Part model, mm, in its own coordinate system. Face numbers are marked on the shaded views. A direction names the side the tool comes from. Give positions to 0.01 mm unless a question says otherwise; leave off trailing zeros. Write each loop counter-clockwise with the first axis right and the second up, starting at its lowest first coordinate (ties: lowest second). Pieces come first, ordered by that corner, then holes.
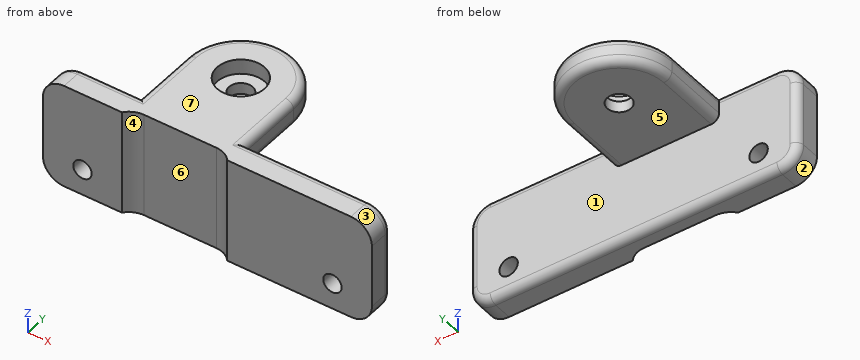
from build123d import *

# Parameters (mm, degrees)
SKETCH2_W                               = 125
SKETCH2_H                               = 40
BOSS_EXTRUDE1_DEPTH                     = 10
BOSS_EXTRUDE2_DEPTH                     = 10
SKETCH4_W                               = 40
SKETCH4_H                               = 3
CUT_EXTRUDE1_DEPTH                      = 80
CBORE_FOR_M8_HEX_HEAD_BOLT1_D           = 9
CBORE_FOR_M8_HEX_HEAD_BOLT1_CBORE_D     = 18.01
CBORE_FOR_M8_HEX_HEAD_BOLT1_CBORE_DEPTH = 5.68
FILLET2_R                               = 8
FILLET3_R                               = 3
F_7_0_7_DIAMETER_HOLE1_D                = 7


with BuildPart() as part:
    # Sketch2 → Boss-Extrude1 (new body)
    with BuildSketch(Plane(origin=(0, 0, 0), x_dir=(1, 0, 0), z_dir=(0, 1, 0))):
        with Locations((62.5, 20)):
            Rectangle(SKETCH2_W, SKETCH2_H)
    extrude(amount=BOSS_EXTRUDE1_DEPTH)

    # Sketch3 → Boss-Extrude2 (add)
    with BuildSketch(Plane.XY):
        with BuildLine():
            Line((30, 35), (30, 0))
            Line((30, 0), (70, 0))
            Line((70, 0), (70, 35))
            ThreePointArc((70, 35), (50, 55), (30, 35))
        make_face()
    extrude(amount=-BOSS_EXTRUDE2_DEPTH)

    # Sketch4 → Cut-Extrude1 (cut)
    with BuildSketch(Plane.XY):
        with Locations((50, 1.5)):
            Rectangle(SKETCH4_W, SKETCH4_H)
    extrude(amount=-CUT_EXTRUDE1_DEPTH, mode=Mode.SUBTRACT)

    # CBORE for M8 Hex Head Bolt1 (through all)
    with Locations(Plane(origin=(50, 35, 0), x_dir=(1, 0, 0), z_dir=(0, 0, 1))):
        with Locations((0, 0)):
            CounterBoreHole(CBORE_FOR_M8_HEX_HEAD_BOLT1_D / 2, CBORE_FOR_M8_HEX_HEAD_BOLT1_CBORE_D / 2, CBORE_FOR_M8_HEX_HEAD_BOLT1_CBORE_DEPTH)

    # Fillet2
    # the kernel refuses this fillet: 8 mm, written as the material it adds along each edge
    with BuildSketch(Plane(origin=(70, 3, 0), x_dir=(-1, 0, 0), z_dir=(0, 0, -1))) as fillet2_piece_1:
        with BuildLine():
            CenterArc((6.244997998, -8), FILLET2_R, 90, 51.317812547)
            Line((0, -3), (0, 0))
            Line((0, 0), (6.244997998, 0))
        make_face()
    extrude(amount=40)
    with BuildSketch(Plane(origin=(30, 3, 0), x_dir=(0, -1, 0), z_dir=(0, 0, -1))) as fillet2_piece_2:
        with BuildLine():
            CenterArc((8, -6.244997998), FILLET2_R, 128.682187453, 51.317812547)
            Line((0, -6.244997998), (0, 0))
            Line((0, 0), (3, 0))
        make_face()
    extrude(amount=40)
    # the kernel refuses this fillet: 8 mm, written as the material it takes off along each edge
    with BuildSketch(Plane(origin=(125, -20, 0), x_dir=(-1, 0, 0), z_dir=(0, 1, 0)), Plane(origin=(125, -20, -40), x_dir=(0, 0, 1), z_dir=(0, 1, 0))) as fillet2_2_piece_1:
        with BuildLine():
            CenterArc((FILLET2_R, -FILLET2_R), FILLET2_R, 90, 90)
            Line((0, -FILLET2_R), (0, 0))
            Line((0, 0), (FILLET2_R, 0))
        make_face()
    extrude(amount=50, mode=Mode.SUBTRACT)
    with BuildSketch(Plane(origin=(0, -20, -40), x_dir=(0, 0, 1), z_dir=(0, 1, 0)), Plane(origin=(0, -20, 0), x_dir=(1, 0, 0), z_dir=(0, 1, 0))) as fillet2_2_piece_2:
        with BuildLine():
            CenterArc((FILLET2_R, FILLET2_R), FILLET2_R, 180, 90)
            Line((0, FILLET2_R), (0, 0))
            Line((0, 0), (FILLET2_R, 0))
        make_face()
    extrude(amount=50, mode=Mode.SUBTRACT)

    # Fillet3
    fillet3_edges = [part.edges().sort_by_distance(p)[0] for p in [
        (93.5, 10, 0),
        (70, 22.5, -10),
        (30, 22.5, -10),
        (70, 22.5, 0),
        (50, 55, 0),
        (30, 22.5, 0),
        (50, 55, -10),
        (125, 10, -20),
        (19, 10, 0),
        (62.5, 10, -40),
        (0, 10, -20),
        (2.343145751, 10, -2.343145751),
        (2.343145751, 10, -37.656854249),
        (122.656854249, 10, -37.656854249),
        (122.656854249, 10, -2.343145751),
    ]]
    fillet(fillet3_edges, radius=FILLET3_R)

    # Ø7.0 (7) Diameter Hole1 (through all)
    with Locations(Plane(origin=(15, 10, -30), x_dir=(0, 0, 1), z_dir=(0, 1, 0))):
        with Locations((0, 0), (0, 95)):
            Hole(F_7_0_7_DIAMETER_HOLE1_D / 2)


solid = part.part
1) Flat gauge pins, fed straight in: P1, Ø14, axis at x = 44.5, z = -20.5, coming from the -Y side; P2, Ø17, axis at x = 37, z = -23.5, coming from the +Y side; P3, Ø3, axis at y = 23.5, z = -5, coming from the +X side. Where does each tip first touch, or does it go through?
Check result:
P1: stops at y = 3
P2: stops at y = 10
P3: stops at x = 70
2) Saw through at C-C (y = 21.5). Write the cut outline in (x, z), and give its area (3 significant figures).
Check result:
outline: (30, -7) arc R3 ccw to (33, -10) - (67, -10) arc R3 ccw to (70, -7) - (70, -3) arc R3 ccw to (67, 0) - (33, 0) arc R3 ccw to (30, -3) - close
area: 392 mm2
3) Drill centre lines: L1, parallel to X at y = 6, z = -30; L2, parallel to Y at x = 50, z = -1.35 (1 decimal); L3, parallel to X at y = 3.5, z = -32. Where is each one in solid material? Low to high.
Check result:
L1: x = 0 to 11.5, 18.5 to 106.5, 113.5 to 125
L2: y = 3 to 26, 44 to 54.5
L3: x = 0 to 12.13, 17.87 to 107.13, 112.87 to 125
4) 3-axis set-ups, long thin cutter, end or side, ignore diameter. For the marked faces 5, 6 and 7: which of +Z, -Z, +X, -X, +Y, -Y reach the whole face in a straight line?
Check result:
face 5: -Z, +X, -X, +Y
face 6: +Z, -Z, -Y
face 7: +Z, +X, -X, +Y, -Y
5) Saw through at B-B (z = -30). Write the cut outline in (x, y) (3 decimals).
Check result:
outline: (0, 0) - (11.5, 0) - (11.5, 10) - (3, 10) arc R3 ccw to (0, 7) - close; (18.5, 0) - (30, 0) arc R8 cw to (36.245, 3) - (63.755, 3) arc R8 cw to (70, 0) - (106.5, 0) - (106.5, 10) - (18.5, 10) - close; (113.5, 0) - (125, 0) - (125, 7) arc R3 ccw to (122, 10) - (113.5, 10) - close
6) Saw through at D-D (z = -19). Write the cut outline in (x, y) (3 decimals).
Check result:
outline: (0, 0) - (30, 0) arc R8 cw to (36.245, 3) - (63.755, 3) arc R8 cw to (70, 0) - (125, 0) - (125, 7) arc R3 ccw to (122, 10) - (3, 10) arc R3 ccw to (0, 7) - close
7) Saw through at A-A (x = 15). Write the cut outline in (y, z).
Check result:
outline: (0, -40) - (7, -40) arc R3 ccw to (10, -37) - (10, -33.5) - (0, -33.5) - close; (0, -26.5) - (10, -26.5) - (10, -3) arc R3 ccw to (7, 0) - (0, 0) - close
8) Mould opens along X. For the marked faces 1, 2, 3 and 4 say: +X half, -X half, draft (parallel to the pull), parting line (faces both ways), or undercut.
Check result:
face 1: draft
face 2: -X half
face 3: +X half
face 4: undercut
